Could you check a few things on this drawing? It's one solid part, dimensions in mm from its lowest x, y, z. Give positions to 0.01 mm unless a question says otherwise; leave off trailing zeros. Order: outer loops, then holes, each group sorted by start corner. A loop starts at its lowest first (then second) coordinate and runs counter-clockwise, first axis right, second up.
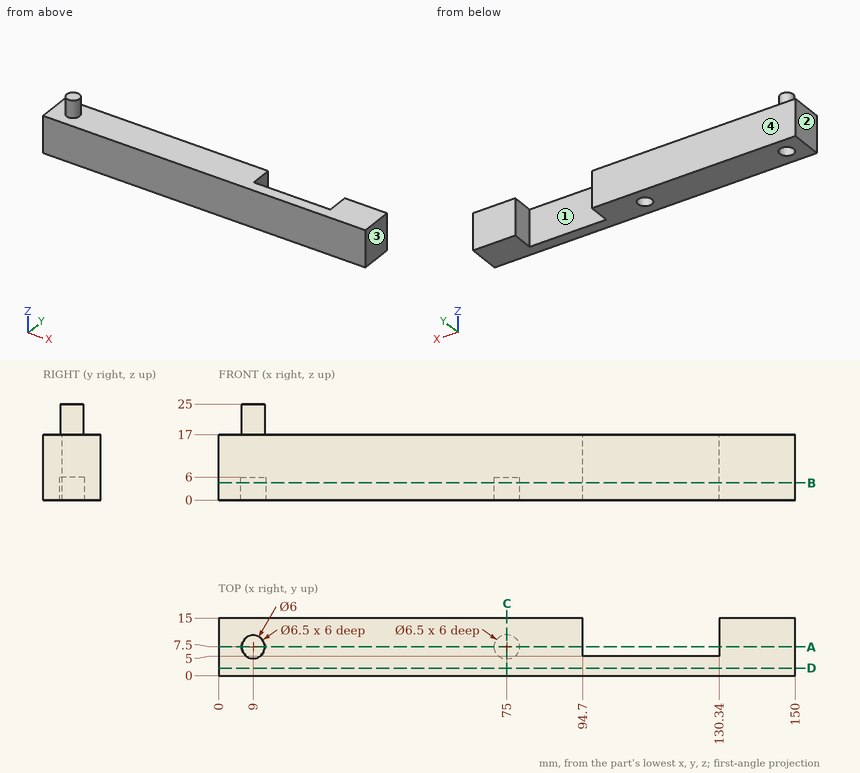
Item 1: Imagine slicing it at C-C on x = 75. List the corners of the cut face in (y, z) for me, then the cut area to 3 significant figures.
Findings:
outline: (0, 0) - (4.25, 0) - (4.25, 6) - (10.75, 6) - (10.75, 0) - (15, 0) - (15, 17) - (0, 17) - close
area: 216 mm2
Item 2: Imagine slicing it at A-A on y = 7.5. List the corners of the cut face in (x, z) for me.
Findings:
outline: (0, 0) - (5.75, 0) - (5.75, 6) - (12.25, 6) - (12.25, 0) - (71.75, 0) - (71.75, 6) - (78.25, 6) - (78.25, 0) - (94.7, 0) - (94.7, 17) - (12, 17) - (12, 25) - (6, 25) - (6, 17) - (0, 17) - close; (130.34, 0) - (150, 0) - (150, 17) - (130.34, 17) - close
Item 3: Please list where these lines run through material, in increasing order: line 1 along Y through (x, z) = (75, 4.3); line 2 along X through (y, z) = (6.75, 10.75); line 3 along Z through (x, y) = (44, 6.25).
Findings:
line 1: y = 0 to 4.25, 10.75 to 15
line 2: x = 0 to 94.7, 130.34 to 150
line 3: z = 0 to 17
Item 4: Imagine slicing it at D-D on y = 2. List the corners of the cut face in (x, z) for me.
Findings:
outline: (0, 0) - (150, 0) - (150, 17) - (0, 17) - close
Item 5: Imagine slicing it at B-B on z = 4.5. List the corners of the cut face in (x, y) for me.
Findings:
outline: (0, 0) - (150, 0) - (150, 15) - (130.34, 15) - (130.34, 5) - (94.7, 5) - (94.7, 15) - (0, 15) - close; hole circle Ø6.5 at (9, 7.5); hole circle Ø6.5 at (75, 7.5)
Item 6: We'd pull the mould along X, two halves only. Please class the marked faces 1, 2, 3 and 4: +X half, -X half, draft (parallel to the pull), parting line (faces both ways), or undercut.
Findings:
face 1: undercut
face 2: -X half
face 3: +X half
face 4: draft
Item 7: For pin 1 (13.5 mm diameter, centred on x = 109, z = 10.5, fed in from +Y); pin 2 (3 mm diameter, centred on x = 7.5, y = 7.5, fed in from -Z); pin 3 (5 mm diameter, centred on x = 90, y = 5, fed in from +Z), each with a flat end and sliding along its axis, tell me the tip position at first contact or that it passes through.
Findings:
pin 1: stops at y = 5
pin 2: stops at z = 6
pin 3: stops at z = 17
